Part model, mm, in its own coordinate system. A direction names the side the tool comes from. Give positions to 0.01 mm unless a question says otherwise; leave off trailing zeros. Order: outer loops, then holes, each group sorted by start corner. A loop starts at its lowest first (then second) coordinate and runs counter-clockwise, first axis right, second up.
1. Probe line 1 (Z direction, x = 0.5, y = 5.75); line 2 (Y direction, x = -4, z = 6); line 3 (X direction, y = 0.5, z = -2). List the from-to ranges inside material, lowest first.
2. Slice it at A-A on z = 0. List the corners of the cut face in (x, y), and give its area (3 significant figures).
3. Slice it at C-C on x = -1.5. Give the number of separate pieces and of enclosed holes in the cut face, and give its area (3 significant figures).
4. Slice it at D-D on z = -10. List the corners of the cut face in (x, y).
5. Mould opens along X. For faces 4 (the flat face through (-9.295, 4.93, -15.384)), 5 (the cylindrical face through (0, 5, -25)), 6 (the cylindrical face through (-1.532, 7.831, 22.697)) say: +X half, -X half, draft (parallel to the pull), parting line (faces both ways), or undercut.
6. Slice it at B-B on y = 1. List the corners of the cut face in (x, z).
7. Which spindle directions (+Z, -Z, +X, -X, +Y, -Y) get a long thin tool onto all of the face, cutting with end or side? Do faces 1 (the cylindrical face through (10.74, 1.01, -2.38)), 2 (the flat face through (-2, 5.6, -21)), 3 (the flat face through (9.445, 4.93, 15.13)). Say none if no direction does.
8. Drop flat-ended pins along their axis: pin 1 Ø6 at (y, z) = (4.5, 7) entering from -X; pin 2 Ø6.5 at (x, z) = (0, 19) entering from +Y; pin 3 Ø3 at (x, y) = (-3, 5.5) entering from -Z. Give the stop position or say it passes through.
from build123d import *

# Parameters (mm, degrees)
BOSS_EXTRUDE1_DEPTH = 10
SKETCH2_R           = 3.99997531
SKETCH2_R_2         = 4
CUT_EXTRUDE1_DEPTH  = 4.4
CUT_EXTRUDE2_REACH  = 32.207
SKETCH3_R           = 2.5
SKETCH4_R           = 11
CUT_EXTRUDE3_DEPTH  = 2
CUT_EXTRUDE4_REACH  = 32.743
SKETCH5_R           = 6
CUT_EXTRUDE5_START  = -2
SKETCH6_R           = 11
CUT_EXTRUDE5_DEPTH  = 2


with BuildPart() as part:
    # Sketch1 → Boss-Extrude1 (new body)
    with BuildSketch(Plane(origin=(0, 0, 0), x_dir=(1, 0, 0), z_dir=(0, 1, 0))):
        with BuildLine():
            Line((-5.103019764, 22.15600792), (-13.605911567, 8.419165811))
            ThreePointArc((-13.605911567, 8.419165811), (-16.001261955, -0.002028565), (-13.605722542, -8.423169172))
            Line((-13.605722542, -8.423169172), (-5.102675537, -22.159834758))
            ThreePointArc((-5.102675537, -22.159834758), (-6.8217e-05, -25.001848451), (5.101614332, -22.158175041))
            Line((5.101614332, -22.158175041), (13.912148597, -7.902456622))
            ThreePointArc((13.912148597, -7.902456622), (15.995958201, 0.300682208), (13.603482502, 8.419167853))
            Line((13.603482502, 8.419167853), (5.100590702, 22.156009965))
            ThreePointArc((5.100590702, 22.156009965), (-0.0012151, 24.998151536), (-5.103019764, 22.15600792))
        make_face()
    extrude(amount=BOSS_EXTRUDE1_DEPTH)

    # Sketch2 → Cut-Extrude1 (cut)
    with BuildSketch(Plane(origin=(0, 10, 0), x_dir=(1, 0, 0), z_dir=(0, 1, 0))):
        with Locations(Location((-0.001213898, 18.998067086, 0), (0, 0, 270))):
            Circle(SKETCH2_R)
        with Locations(Location((-6.8217e-05, -19.001848451, 0), (0, 0, 270))):
            Circle(SKETCH2_R_2)
    extrude(amount=-CUT_EXTRUDE1_DEPTH, mode=Mode.SUBTRACT)

    # Sketch3 → Cut-Extrude2 (cut, up to next)
    with BuildSketch(Plane(origin=(0, 5.6, 0), x_dir=(1, 0, 0), z_dir=(0, 1, 0)), mode=Mode.PRIVATE) as cut_extrude2_sk1:
        with Locations(Location((-0.001213898, 18.998067086, 0), (0, 0, 270))):
            Circle(SKETCH3_R)
    cut_extrude2_tool1 = extrude(cut_extrude2_sk1.sketch, amount=-CUT_EXTRUDE2_REACH, mode=Mode.PRIVATE) & part.part
    # Sketch3 → Cut-Extrude2 (cut, up to next)
    with BuildSketch(Plane(origin=(0, 5.6, 0), x_dir=(1, 0, 0), z_dir=(0, 1, 0)), mode=Mode.PRIVATE) as cut_extrude2_sk2:
        with Locations(Location((-6.8217e-05, -19.001848451, 0), (0, 0, 270))):
            Circle(SKETCH3_R)
    cut_extrude2_tool2 = extrude(cut_extrude2_sk2.sketch, amount=-CUT_EXTRUDE2_REACH, mode=Mode.PRIVATE) & part.part
    add(cut_extrude2_tool1.solids().sort_by_distance((-0.001214, 5.6, -18.998067))[0], mode=Mode.SUBTRACT)
    add(cut_extrude2_tool2.solids().sort_by_distance((-6.8e-05, 5.6, 19.001848))[0], mode=Mode.SUBTRACT)

    # Sketch4 → Cut-Extrude3 (cut)
    with BuildSketch(Plane(origin=(0, 10, 0), x_dir=(1, 0, 0), z_dir=(0, 1, 0))):
        with Locations(Location((0, 0, 0), (0, 0, 270))):
            Circle(SKETCH4_R)
    extrude(amount=-CUT_EXTRUDE3_DEPTH, mode=Mode.SUBTRACT)

    # Sketch5 → Cut-Extrude4 (cut, up to next)
    with BuildSketch(Plane(origin=(0, 8, 0), x_dir=(1, 0, 0), z_dir=(0, 1, 0)), mode=Mode.PRIVATE) as cut_extrude4_sk1:
        with Locations(Location((0, 0, 0), (0, 0, 270))):
            Circle(SKETCH5_R)
    cut_extrude4_tool1 = extrude(cut_extrude4_sk1.sketch, amount=-CUT_EXTRUDE4_REACH, mode=Mode.PRIVATE) & part.part
    add(cut_extrude4_tool1.solids().sort_by_distance((0, 8, 0))[0], mode=Mode.SUBTRACT)

    # Sketch6 → Cut-Extrude5 (cut)
    with BuildSketch(Plane.XZ.offset(CUT_EXTRUDE5_START)):
        with Locations(Location((0, 0, 0), (0, 0, 90))):
            Circle(SKETCH6_R)
    extrude(amount=CUT_EXTRUDE5_DEPTH, mode=Mode.SUBTRACT)


solid = part.part
Data:
1. line 1: z = -24.98 to -22.97, -15.03 to -5.98, 5.98 to 15.03, 22.97 to 24.98
1. line 2: y = 2 to 8
1. line 3: x = -15.88 to -10.82, 10.82 to 15.87
2. outline: (-16, 0) - (-11, 0) - (-11, 2) - (-6, 2) - (-6, 8) - (-11, 8) - (-11, 10) - (-16, 10) - close; (6, 2) - (11, 2) - (11, 0) - (16, 0) - (16, 10) - (11, 10) - (11, 8) - (6, 8) - close
2. area: 160 mm2
3. separate pieces: 4
3. enclosed holes: 0
3. area: 229 mm2
4. outline: (-12.63, 0) - (-4.58, 0) - (-4.58, 2) - (4.58, 2) - (4.58, 0) - (12.62, 0) - (12.62, 10) - (4.58, 10) - (4.58, 8) - (-4.58, 8) - (-4.58, 10) - (-12.63, 10) - close
5. face 4: -X half
5. face 5: parting line
5. face 6: undercut
6. outline: (-13.61, -8.42) - (-5.1, -22.16) arc R6 ccw to (5.1, -22.16) - (13.6, -8.42) arc R16 ccw to (13.91, 7.9) - (5.1, 22.16) arc R6 ccw to (-5.1, 22.16) - (-13.61, 8.42) arc R16 ccw to start; hole circle Ø22 at (0, 0); hole circle Ø5 at (0, -19); hole circle Ø5 at (0, 19)
7. face 1: -Y
7. face 2: +Y
7. face 3: +Z, +X, +Y, -Y
8. pin 1: stops at x = -15.49
8. pin 2: stops at y = 5.6
8. pin 3: stops at z = -24.81
